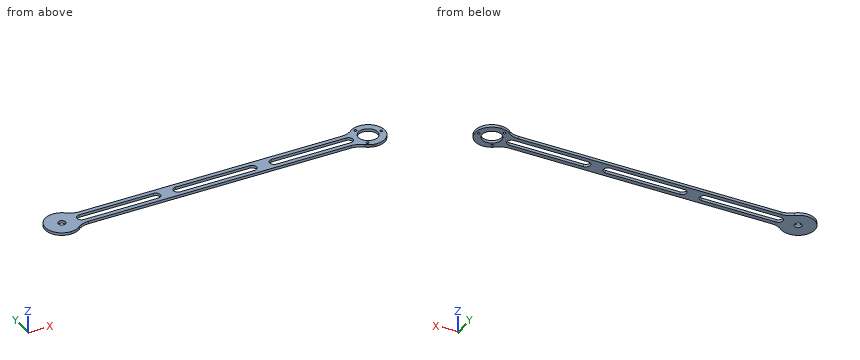
```python
from build123d import *

# Parameters (mm, degrees)
SKETCH1_R               = 4.075
SKETCH1_R_2             = 11.075
BOSS_EXTRUDE1_DEPTH     = 1.5
CUT_EXTRUDE2_DEPTH      = 370.491880831
CUT_EXTRUDE2_DEPTH_BACK = 370.491880831
SKETCH3_R               = 1.5
CUT_EXTRUDE3_DEPTH      = 370.491880831
CUT_EXTRUDE3_DEPTH_BACK = 370.491880831


with BuildPart() as part:
    # Sketch1 → Boss-Extrude1 (new, symmetric)
    with BuildSketch(Plane.XY):
        with BuildLine():
            Line((24.919871589, 10), (325.080128411, 10))
            ThreePointArc((325.080128411, 10), (331.873790616, 11.189201137), (337.859549739, 14.615384615))
            ThreePointArc((337.859549739, 14.615384615), (343.546020905, 17.870258919), (350, 19))
            ThreePointArc((350, 19), (369, 0), (350, -19))
            ThreePointArc((350, -19), (343.546020905, -17.870258919), (337.859549739, -14.615384615))
            ThreePointArc((337.859549739, -14.615384615), (331.873790616, -11.189201137), (325.080128411, -10))
            Line((325.080128411, -10), (24.919871589, -10))
            ThreePointArc((24.919871589, -10), (18.126209384, -11.189201137), (12.140450261, -14.615384615))
            ThreePointArc((12.140450261, -14.615384615), (6.453979095, -17.870258919), (0, -19))
            ThreePointArc((0, -19), (-19, 0), (0, 19))
            ThreePointArc((0, 19), (6.453979095, 17.870258919), (12.140450261, 14.615384615))
            ThreePointArc((12.140450261, 14.615384615), (18.126209384, 11.189201137), (24.919871589, 10))
        make_face()
        Circle(SKETCH1_R, mode=Mode.SUBTRACT)
        with Locations((350, 0)):
            Circle(SKETCH1_R_2, mode=Mode.SUBTRACT)
    extrude(amount=BOSS_EXTRUDE1_DEPTH, both=True)

    # Sketch3 → Cut-Extrude2 (cut, two sides: drawn at the far end of the back side and taken through both)
    with BuildSketch(Plane.XY.offset(-CUT_EXTRUDE2_DEPTH_BACK)):
        with Locations((365, 0)):
            Circle(SKETCH3_R)
        with Locations((342.5, -12.990381057)):
            Circle(SKETCH3_R)
        with Locations((342.5, 12.990381057)):
            Circle(SKETCH3_R)
    extrude(amount=CUT_EXTRUDE2_DEPTH + CUT_EXTRUDE2_DEPTH_BACK, mode=Mode.SUBTRACT)

    # Sketch4 → Cut-Extrude3 (cut, two sides: drawn at the far end of the back side and taken through both)
    with BuildSketch(Plane.XY.offset(-CUT_EXTRUDE3_DEPTH_BACK)):
        with BuildLine():
            Line((22.5, 5), (107.5, 5))
            ThreePointArc((107.5, 5), (112.5, 0), (107.5, -5))
            Line((107.5, -5), (22.5, -5))
            ThreePointArc((22.5, -5), (17.5, 0), (22.5, 5))
        make_face()
        with BuildLine():
            Line((132.5, 5), (217.5, 5))
            ThreePointArc((217.5, 5), (222.5, 0), (217.5, -5))
            Line((217.5, -5), (132.5, -5))
            ThreePointArc((132.5, -5), (127.5, 0), (132.5, 5))
        make_face()
        with BuildLine():
            Line((242.5, 5), (327.5, 5))
            ThreePointArc((327.5, 5), (332.5, 0), (327.5, -5))
            Line((327.5, -5), (242.5, -5))
            ThreePointArc((242.5, -5), (237.5, 0), (242.5, 5))
        make_face()
    extrude(amount=CUT_EXTRUDE3_DEPTH + CUT_EXTRUDE3_DEPTH_BACK, mode=Mode.SUBTRACT)


solid = part.part
```
Could you check a few things on this model? Use its own coordinates, in mm. Round coordinates to 2 decimals unless told otherwise and drop trailing zeros. Write each loop counter-clockwise with the first axis right and the second up, starting at its lowest first coordinate (ties: lowest second). Pieces come first, ordered by that corner, then holes. Notation, with made-up numbers: M 46,-10.75 L 95,-10.75 A13 ccw 95,13.25 Z; hole C -17,70 d4. An arc over 180 degrees is marked long. Write each question's results on one line, items separated by ' | '. Start each with the question number.
1. Imagine slicing it at A-A on x = 249.5. List the corners of the cut face in (y, z) for me.
2. I'm going to push flat-ended pins straight in: pin 1 Ø2.5 at (x, y) = (365, 0) entering from -Z; pin 2 Ø1 at (x, z) = (205.5, 0) entering from +Y; pin 3 Ø3.5 at (x, y) = (342.5, 12.99) entering from +Z; pin 4 Ø0.9 at (x, z) = (159.5, -0.5) entering from -Y. Where does each tip first touch, or does it pass through?
3. Imagine slicing it at B-B on z = 0.8. Count the separate pieces of the cut face and the enclosed holes in it, and give its area (3 significant figures).
4. I need wall thicknesses on L1, parallel to Y at x = 204.5, z = 1.15; L2, parallel to X at y = 3, z = -0.6; L3, parallel to Y at x = 350, z = 0.85 (3 decimals). Which ranges of each line are inside material? Lowest first, please. Write a range as from..to.
Result sheet:
1) outline: M -10,-1.5 L -5,-1.5 L -5,1.5 L -10,1.5 Z; M 5,-1.5 L 10,-1.5 L 10,1.5 L 5,1.5 Z
2) pin 1: passes through | pin 2: stops at y = 10 | pin 3: stops at z = 1.5 | pin 4: stops at y = -10
3) separate pieces: 1 | enclosed holes: 8 | area: 5,330 mm^2
4) L1: y = -10..-5, 5..10 | L2: x = -18.76..-2.76, 2.76..18.5, 111.5..128.5, 221.5..238.5, 331.5..339.34, 360.66..368.76 | L3: y = -19..-11.075, 11.075..19
